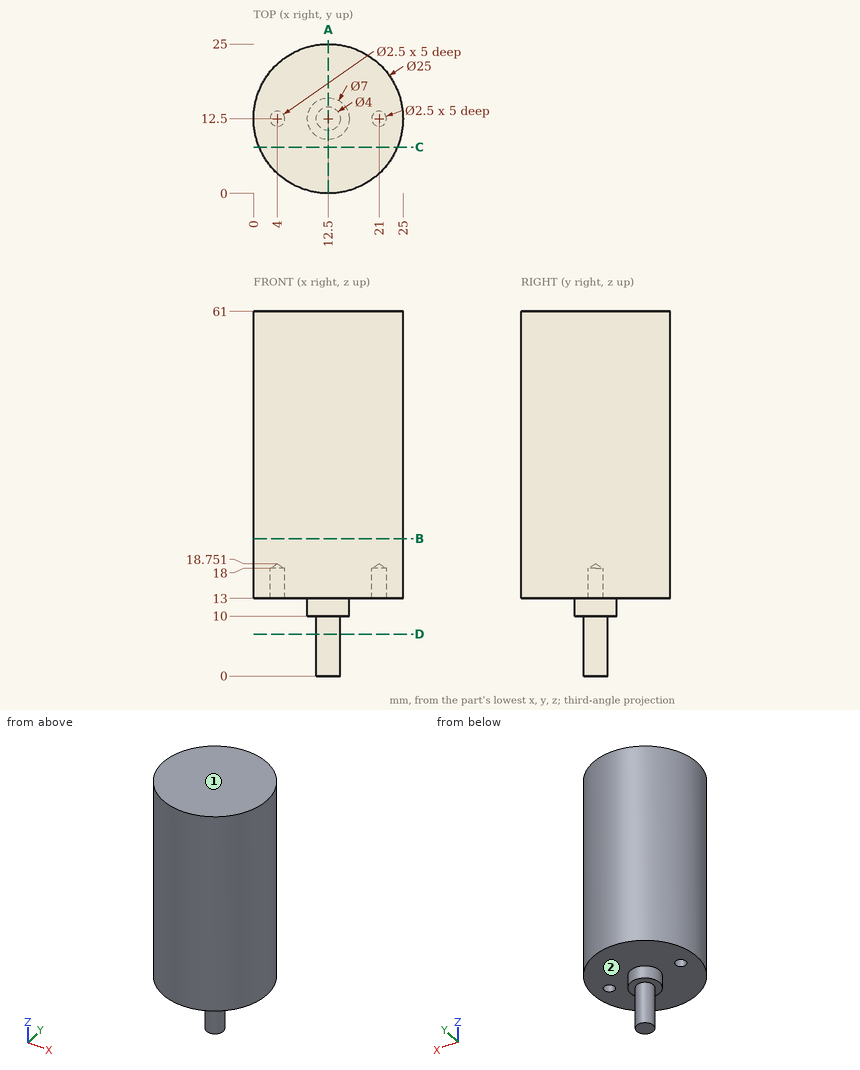
Verification items for this drawing (mm, ordinates from the low corner). A direction names the side the tool comes from. Give positions to 0.01 mm unless a question says otherwise; leave off trailing zeros. Write each loop counter-clockwise with the first axis right and the second up, starting at its lowest first coordinate (ties: lowest second). Pieces come first, ordered by that corner, then holes.
1) Section check D-D, the plane z = 7. Record the boundary of the cut face in (x, y), and give its area (3 significant figures).
2) Section check A-A, the plane x = 12.5. Record the boundary of the cut face in (y, z), and give its area (3 significant figures).
3) Gauge pin test, flat ends, axial feed: pin 1 (5 mm diameter, centred on x = 20.5, z = 32, fed in from -Y) (3 decimals); pin 2 (7.5 mm diameter, centred on x = 17.5, y = 11.5, fed in from -Z); pin 3 (1 mm diameter, centred on x = 22.5, y = 11.5, fed in from -Z); pin 4 (3 mm diameter, centred on x = 16.5, z = 21, fed in from +Y). Record the tip position at first contact, or that the pin passes through.
4) Access from +Z, -Z, +X, -X, +Y, -Y to the whole of each face (thin tool, end or side, straight path). Record for the marked faces 1 and 2.
5) Section check B-B, the plane z = 23. Record the boundary of the cut face in (x, y), and give its area (3 significant figures).
6) Section check C-C, the plane y = 7.75. Record the boundary of the cut face in (x, z).
7) Material ranges on L1, parallel to Z at x = 10, y = 8.75; L2, parallel to Y at x = 13, z = 54.5; L3, parallel to X at y = 4.25, z = 46, recorded low to high.
Computed:
1. outline: circle Ø4 at (12.5, 12.5)
1. area: 12.6 mm2
2. outline: (0, 13) - (9, 13) - (9, 10) - (10.5, 10) - (10.5, 0) - (14.5, 0) - (14.5, 10) - (16, 10) - (16, 13) - (25, 13) - (25, 61) - (0, 61) - close
2. area: 1,260 mm2
3. pin 1: stops at y = 1.275
3. pin 2: stops at z = 0
3. pin 3: stops at z = 13
3. pin 4: stops at y = 24.75
4. face 1: +Z, +X, -X, +Y, -Y
4. face 2: -Z
5. outline: circle Ø25 at (12.5, 12.5)
5. area: 491 mm2
6. outline: (0.94, 13) - (24.06, 13) - (24.06, 61) - (0.94, 61) - close
7. L1: z = 13 to 61
7. L2: y = 0.01 to 24.99
7. L3: x = 3.11 to 21.89
